Check sheet for the drawn part. Datum: minimum x, y, z corner. Units: mm. Round coordinates to 2 decimals unless told otherwise and drop trailing zeros. Use CSV: the item, a comma, the result in double quotes. Start each with the question number.
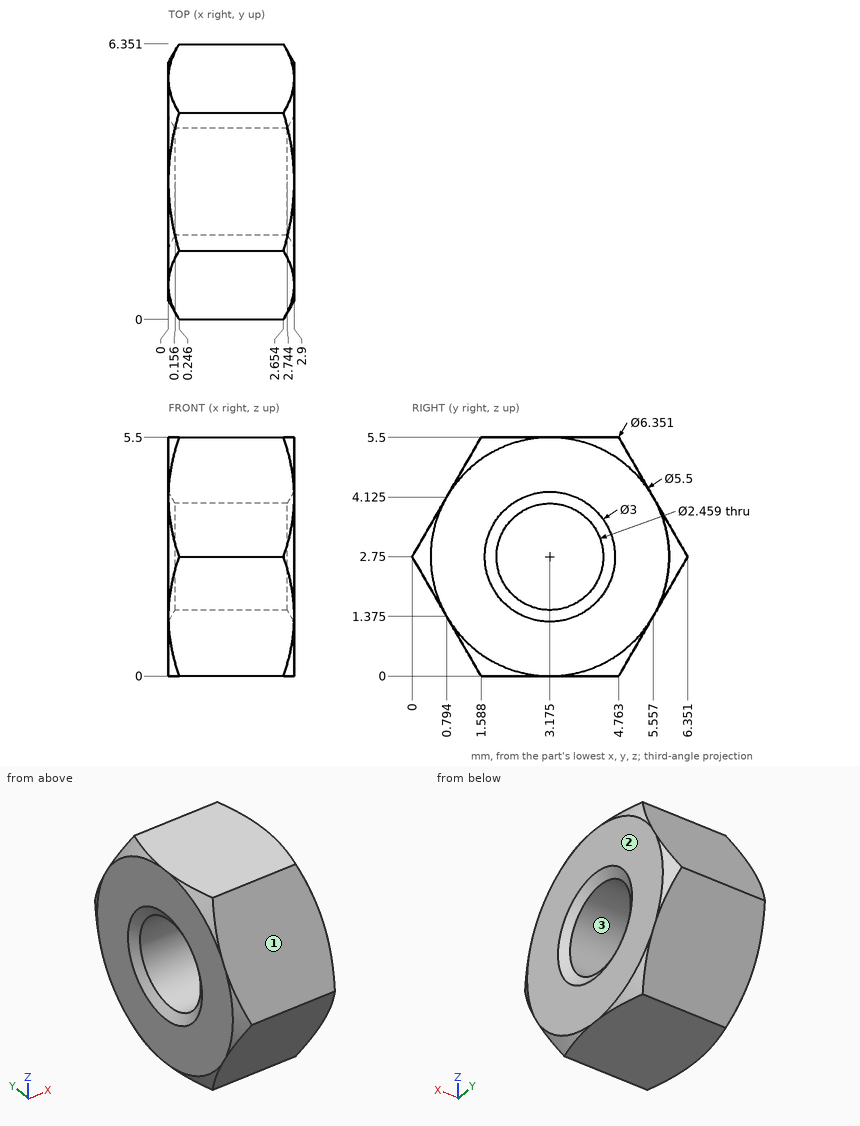
Q1. Depth check by flat-ended pin: pin 1 Ø1 at (x, y) = (2.5, 5.5) entering from +Z. Enter the tip coordinate at first touch or a pass-through.
Q2. Release check for a two-part mould opening along Z. For the marked faces 1, 2 and 3 record: +Z half, -Z half, draft (parallel to the pull), parting line (faces both ways), or undercut.
Q3. Thickness scan on L1, parallel to Z at x = 0.25, y = 2.25; L2, parallel to Z at x = 1.55, y = 2.75 (1 decimal); L3, parallel to Y at x = 0.2, z = 3.25. Record the ranges inside material, lowest first. Write a range as from..to.
Answer list:
1,pin 1,"stops at z = 5.09"
2,face 1,"+Z half"
2,face 2,"draft"
2,face 3,"undercut"
3,L1,"z = 0..1.94, 3.56..5.5"
3,L2,"z = 0..1.6, 3.9..5.5"
3,L3,"y = 0.29..2.05, 4.3..6.06"
